Print and shaded views of the part. All mm, measured from the part's lowest x, y and z. Give positions to 0.01 mm unless a question says otherwise; leave off trailing zeros. Loops run counter-clockwise (first coordinate to the right, second up) from the corner with the lowest first, then second, coordinate; pieces in that order, holes last. Notation, with made-up numbers: M 56,37.5 L 98,37.5 A22 cw 98,55.5 Z; hole C -20.5,19.25 d7. An arc over 180 degrees is marked long. Answer in a Markdown table with one row per item.
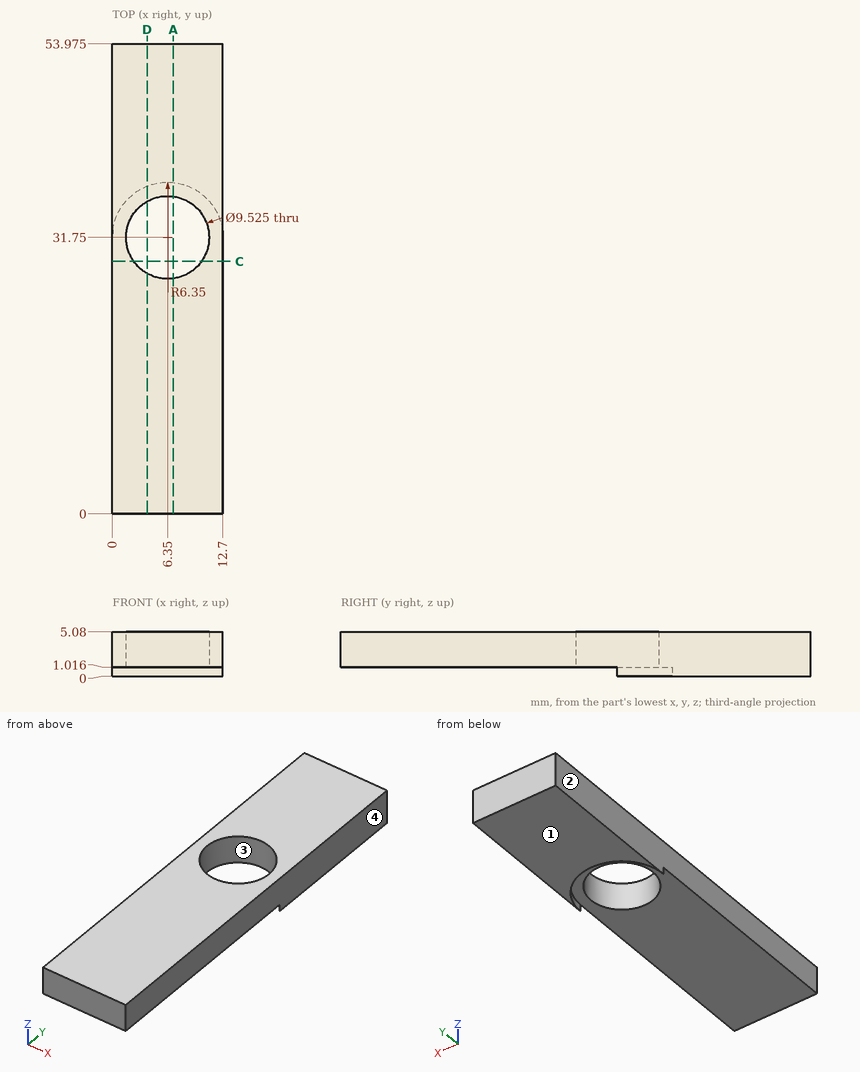
(1) Flat gauge pins, fed straight in: P1, Ø4, axis at x = 5, y = 14, coming from the -Z side; P2, Ø5.5, axis at x = 6.35, y = 31.75, coming from the +Z side. Where does each tip first touch, or does it go through?
Established:
| item | result |
|---|---|
| P1 | stops at z = 1.02 |
| P2 | passes through |
(2) Wall check: L1, parallel to Y at x = 6.35, z = 1.95 (1 decimal); L2, parallel to Z at x = 8.5, y = 4; L3, parallel to X at y = 33, z = 1.6. Give the ranges that are in metal, low to high.
Established:
| item | result |
|---|---|
| L1 | y = 0 to 27, 36.5 to 54 |
| L2 | z = 1.02 to 5.08 |
| L3 | x = 0 to 1.75, 10.95 to 12.7 |
(3) Saw through at A-A, the plane x = 7. Give the cut face in (y, z) (3 decimals).
Established:
| item | result |
|---|---|
| outline | M 0,1.016 L 27.032,1.016 L 27.032,5.08 L 0,5.08 Z; M 36.468,1.016 L 38.067,1.016 L 38.067,0 L 53.975,0 L 53.975,5.08 L 36.468,5.08 Z |
(4) Saw through at C-C, the plane y = 29. Give the cut face in (x, z).
Established:
| item | result |
|---|---|
| outline | M 0,1.02 L 2.46,1.02 L 2.46,5.08 L 0,5.08 Z; M 10.24,1.02 L 12.7,1.02 L 12.7,5.08 L 10.24,5.08 Z |
(5) Mould opens along X. For the marked faces 1, 2, 3 and 4 say: pulls with the +X half, pulls with the -X half, needs draft (parallel to the pull), parting line crosses it, or undercut.
Established:
| item | result |
|---|---|
| face 1 | needs draft |
| face 2 | pulls with the -X half |
| face 3 | undercut |
| face 4 | pulls with the +X half |
(6) Saw through at D-D, the plane x = 4. Give the cut face in (y, z) (3 decimals), and give its area (3 significant figures).
Established:
| item | result |
|---|---|
| outline | M 0,1.016 L 27.608,1.016 L 27.608,5.08 L 0,5.08 Z; M 35.892,1.016 L 37.649,1.016 L 37.649,0 L 53.975,0 L 53.975,5.08 L 35.892,5.08 Z |
| area | 202 mm2 |
